Can you work these out from the model? Positions are in its coordinate system, mm. Face numbers are marked on the shaded views. A direction names the side the tool comes from. Give positions to 0.01 mm unless a question says otherwise; leave off trailing zeros. Loops run counter-clockwise (first coordinate to the right, second up) from the corner with the lowest first, then second, coordinate; pieces in that order, holes last. Notation, with made-up numbers: M 2.25,66.5 L 55.25,66.5 A8 ccw 55.25,74.5 Z; hole C -22,43.25 d7. An arc over 180 degrees is marked long. Put each result on its own line as item: value. Start each with the question number.
1) Imagine slicing it at B-B (y = 0). Write out the boundary of the cut face in (x, z).
2) Imagine slicing it at C-C (z = 12.5). Write out the boundary of the cut face in (x, y), then the cut area to 3 significant figures.
3) Please list where these lines run through material, in increasing order: line 1 along Y through (x, z) = (6.25, 0); line 2 along Y through (x, z) = (12.3, 0); line 3 along Y through (x, z) = (7.5, 10). Write a range as from..to.
4) For the marked faces 4, 5, 6, 7 and 8, which set-ups out of +Z, -Z, +X, -X, +Y, -Y let a thin tool reach every point of the face, with its end or its side?
5) For P1, Ø2, axis at x = 2.5, y = -4.5, coming from the -Z side, with a flat end and sliding along its axis, tell me the tip position at first contact or that it passes through.
6) Imagine slicing it at A-A (z = 0). Write out the boundary of the cut face in (x, y), then the cut area to 3 significant figures.
7) If we mould it in two halves opening along Y, with no side actions, what happens to the marked faces 1, 2 and 3? For each: +Y half, -Y half, draft (parallel to the pull), parting line (faces both ways), or undercut.
from build123d import *

# Parameters (mm, degrees)
BASPROSKE_W             = 8
BASPROSKE_H             = 15
TOOTHCUT_DEPTH          = 23.671568097
TEETHCUTS_COUNT         = 18
TEETHCUTS_ANGLE         = 340
BORSKE_R                = 0.4
BORE_DEPTH              = 50.0000508
ESQUISSE1_R             = 5
BOSS_EXTRU_1_DEPTH      = 5
ESQUISSE2_R             = 2.85
ENL_V_MAT_EXTRU_1_DEPTH = 3
ESQUISSE3_R             = 1
ENL_V_MAT_EXTRU_2_DEPTH = 24.345559985


with BuildPart() as part:
    # BasProSke → Base-Revolve (revolve)
    with BuildSketch(Plane(origin=(0, 0, 0), x_dir=(1, 0, 0), z_dir=(0, 1, 0)), mode=Mode.PRIVATE) as base_revolve_sk:
        with Locations((4, 7.5)):
            Rectangle(BASPROSKE_W, BASPROSKE_H)
    revolve(base_revolve_sk.sketch.rotate(Axis((-10, 0, 0), (1, 0, 0)), 180), axis=Axis((-10, 0, 0), (1, 0, 0)))

    # TooCutSke → ToothCut (cut, through all)
    with BuildSketch(Plane(origin=(0, 0, 0), x_dir=(0, 0, -1), z_dir=(1, 0, 0))):
        with BuildLine():
            ThreePointArc((0.759974923, 11.599129886), (0, 11.624), (-0.759974923, 11.599129886))
            ThreePointArc((-0.759974923, 11.599129886), (-1.229186471, 13.354767823), (-2.254227748, 14.855339189))
            ThreePointArc((-2.254227748, 14.855339189), (0, 15.0254), (2.254227748, 14.855339189))
            ThreePointArc((2.254227748, 14.855339189), (1.229186471, 13.354767823), (0.759974923, 11.599129886))
        make_face()
    toothcut = extrude(amount=TOOTHCUT_DEPTH, mode=Mode.SUBTRACT)

    # TeethCuts: ToothCut ×18 about axis
    teethcuts_axis = Axis((-10, 0, 0), (1, 0, 0))
    for i in range(1, TEETHCUTS_COUNT):
        add(toothcut.rotate(teethcuts_axis, i * TEETHCUTS_ANGLE / (TEETHCUTS_COUNT - 1)), mode=Mode.SUBTRACT)

    # BorSke → Bore (cut, symmetric)
    with BuildSketch(Plane(origin=(0, 0, 0), x_dir=(0, 0, -1), z_dir=(1, 0, 0))):
        with Locations(Location((0, 0, 0), (0, 0, 180))):
            Circle(BORSKE_R)
    extrude(amount=BORE_DEPTH, both=True, mode=Mode.SUBTRACT)

    # Esquisse1 → Boss.-Extru.1 (add)
    with BuildSketch(Plane(origin=(8, 0, 0), x_dir=(0, 0, -1), z_dir=(1, 0, 0))):
        with Locations(Location((0, 0, 0), (0, 0, 180))):
            Circle(ESQUISSE1_R)
    extrude(amount=BOSS_EXTRU_1_DEPTH)

    # Esquisse2 → Enlèv. mat.-Extru.1 (cut)
    with BuildSketch(Plane(origin=(13, 0, 0), x_dir=(0, 0, -1), z_dir=(1, 0, 0))):
        Circle(ESQUISSE2_R)
    extrude(amount=-ENL_V_MAT_EXTRU_1_DEPTH, mode=Mode.SUBTRACT)

    # Esquisse3 → Enlèv. mat.-Extru.2 (cut, through all)
    with BuildSketch(Plane(origin=(10, 0, 0), x_dir=(0, 0, -1), z_dir=(1, 0, 0))):
        Circle(ESQUISSE3_R)
    extrude(amount=-ENL_V_MAT_EXTRU_2_DEPTH, mode=Mode.SUBTRACT)


solid = part.part
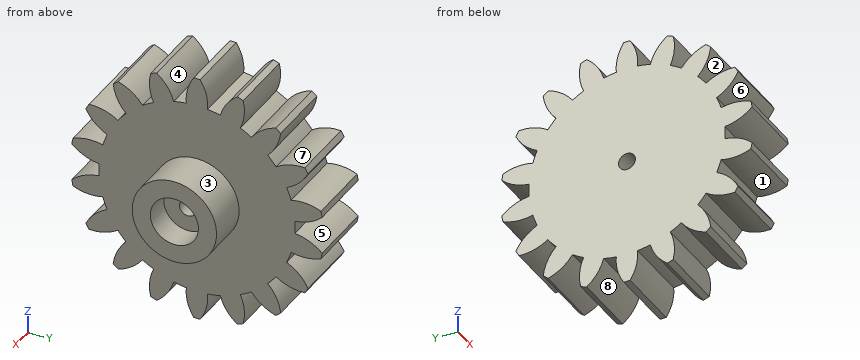
Recorded:
1. outline: M 0,-15 L 8,-15 L 8,-5 L 13,-5 L 13,-2.85 L 10,-2.85 L 10,-1 L 0,-1 Z; M 0,1 L 10,1 L 10,2.85 L 13,2.85 L 13,5 L 8,5 L 8,15 L 0,15 Z
2. outline: M 0,-5.63 L 8,-5.63 L 8,-3.26 L 0,-3.26 Z; M 0,-1.26 L 8,-1.26 L 8,1.26 L 0,1.26 Z; M 0,3.26 L 8,3.26 L 8,5.63 L 0,5.63 Z
2. area: 58.2 mm²
3. line 1: -11.62..-1, 1..11.62
3. line 2: -5..-2.85, 2.85..5
3. line 3: -9.64..-6.71, -5.93..5.93, 6.71..9.64
4. face 4: +Z, +X, -X
4. face 5: +X, -X, +Y
4. face 6: +X, -X, -Y
4. face 7: +X, -X
4. face 8: -Z, +X, -X
5. P1: z = -14.22
6. outline: M 0,-11.62 L 8,-11.62 L 8,-5 L 13,-5 L 13,-2.85 L 10,-2.85 L 10,-1 L 0,-1 Z; M 0,1 L 10,1 L 10,2.85 L 13,2.85 L 13,5 L 8,5 L 8,11.62 L 0,11.62 Z
6. area: 199 mm²
7. face 1: undercut
7. face 2: -Y half
7. face 3: parting line
